Source: CAD feature listing. Evaluate the final solid. Frame: model axes, mm. A direction names the side the tool comes from. Coordinates: 2 decimals unless noted, no trailing zeros. Order: outer loops, then holes, each group sorted by start corner. A loop starts at its lowest first (then second) coordinate and runs counter-clockwise, first axis right, second up. Notation, with made-up numbers: (-12, -8.5) -> (9, -8.5) arc R12 cw to (9, -1.5) -> close; hole circle Ø9 at (55, 40.25). An arc over 180 degrees is marked (long way). Write each question's results on one line, items separated by ' | '. Start each with the question number.
Autodesk Inventor part; units mm, degrees
sketch "Sketch1" plane through (0, 0, 0) normal (0, 0, 1) x (1, 0, 0)
  line L0 (-120, 6.5) -> (120, 6.5)
  line L1 (120, 6.5) -> (120, -6.5)
  line L2 (120, -6.5) -> (-120, -6.5)
  line L3 (-120, -6.5) -> (-120, 6.5)
  line L4 (-120, 6.5) -> (120, -6.5) construction
  line L5 (120, 6.5) -> (-120, -6.5) construction
  point P0 (0, 0)
  point P1 (0, 0)
  dimension "d0" = 240
  dimension "d1" = 13
extrude "Extrusion1" add sketch "Sketch1" along normal mid plane 8
sketch "Sketch2" plane through (0, 0, 4) normal (0, 0, 1) x (1, 0, 0)
  circle A0 centre (-109, 0) radius 1.5
  circle A1 centre (-95, 0) radius 1.5
  circle A2 centre (95, 0) radius 1.5
  circle A3 centre (109, 0) radius 1.5
  point P0 (0, 0)
extrude "Extrusion2" cut sketch "Sketch2" against normal through all
sketch "Sketch3" plane through (0, 0, 4) normal (0, 0, 1) x (1, 0, 0)
  line L0 (-95, 0) -> (-109, 0) construction
  circle A0 centre (-95, 0) radius 1.5
  circle A1 centre (-109, 0) radius 1.5
  line L1 (-91, 4.5) -> (-113, 4.5)
  line L2 (-113, 4.5) -> (-113, -4.5)
  line L3 (-113, -4.5) -> (-91, -4.5)
  line L4 (-91, -4.5) -> (-91, 4.5)
  line L5 (-91, 4.5) -> (-113, -4.5) construction
  line L6 (-113, 4.5) -> (-91, -4.5) construction
  circle A2 centre (109, 0) radius 1.5
  circle A3 centre (95, 0) radius 1.5
  line L7 (109, 0) -> (95, 0) construction
  line L8 (113, 4.5) -> (91, 4.5)
  line L9 (91, 4.5) -> (91, -4.5)
  line L10 (91, -4.5) -> (113, -4.5)
  line L11 (113, -4.5) -> (113, 4.5)
  line L12 (113, 4.5) -> (91, -4.5) construction
  line L13 (91, 4.5) -> (113, -4.5) construction
  point P0 (0, 0)
  point P1 (-102, 0)
  point P2 (-102, 0)
  point P3 (102, 0)
  point P4 (102, 0)
  dimension "d9" = 22
  dimension "d10" = 9
extrude "Extrusion3" cut sketch "Sketch3" against normal blind 3
properties part number "conector_eixos_001" material "ABS Plastic"
(1) Section A-A on z = 2.5. Return the cut outline in (x, y).
(2) Reachability of faces 1 (the flat face through (120, 0, 0)), 2 (the flat face through (-102, 0, 1)) from +Z, -Z, +X, -X, +Y, -Y: full face, straight path, thin tool, end or side. Return the list, or none.
(3) Draft query along Y for faces 3 (the flat face through (102, 0, 1)), 4 (the flat face through (2, -6.5, 0)), 5 (the flat face through (-2, 0, 4)), 6 (the flat face through (-2, 6.5, 0)). Return one class per face: released by +Y, released by -Y, zero draft, split by the parting line, or undercut.
(4) First-contact query: P1, Ø4.5, axis at x = 101, y = -2, coming from the +Z side. Flat tip, straight axial feed; report the tip coordinate or a pass-through.
(5) Line query: L1, parallel to Y at x = 95, z = -1.35; L2, parallel to X at y = 3.75, z = 2.5; L3, parallel to Z at x = 106, y = -0.25. Output: solid intervals per line, ascending.
Results list:
1) outline: (-120, -6.5) -> (120, -6.5) -> (120, 6.5) -> (-120, 6.5) -> close; hole (-113, -4.5) -> (-91, -4.5) -> (-91, 4.5) -> (-113, 4.5) -> close; hole (91, -4.5) -> (113, -4.5) -> (113, 4.5) -> (91, 4.5) -> close
2) face 1: +Z, -Z, +X, +Y, -Y | face 2: +Z
3) face 3: undercut | face 4: released by -Y | face 5: zero draft | face 6: released by +Y
4) P1: stops at z = 1
5) L1: y = -6.5 to -1.5, 1.5 to 6.5 | L2: x = -120 to -113, -91 to 91, 113 to 120 | L3: z = -4 to 1
